CAD build for the part. Positions are in the model's coordinates, mm. A direction names the side the tool comes from. Round coordinates to 2 decimals unless told otherwise and drop trailing zeros. Loops run counter-clockwise (first coordinate to the right, second up) from the corner with the lowest first, then second, coordinate; pieces in that order, holes last. Notation, with made-up numbers: (37, 84) - (60, 84) arc R14 ccw to (60, 105) - close; hole circle Ø7 at (-9, 60). An arc over 180 degrees is marked (long way). One line per question, with ' | ' between items.
```python
from build123d import *

# Parameters (mm, degrees)
SKETCH2_W           = 75
SKETCH2_H           = 48
BOSS_EXTRUDE1_DEPTH = 7.75
CUT_EXTRUDE4_DEPTH  = 12.5
SKETCH12_W          = 50
SKETCH12_H          = 38
CUT_EXTRUDE5_DEPTH  = 7.75
SKETCH13_R          = 0.625
CUT_EXTRUDE6_DEPTH  = 47.006113724
FILLET4_R           = 3
SKETCH14_W          = 2
SKETCH14_H          = 5
BOSS_EXTRUDE2_DEPTH = 2
SKETCH16_R          = 1.25
CUT_EXTRUDE9_DEPTH  = 1
SKETCH18_R          = 5
CUT_EXTRUDE10_DEPTH = 3
SKETCH19_R          = 7.5
CUT_EXTRUDE11_DEPTH = 0.5


with BuildPart() as part:
    # Sketch2 → Boss-Extrude1 (new, symmetric)
    with BuildSketch(Plane.XY):
        with Locations((0, 1.5)):
            Rectangle(SKETCH2_W, SKETCH2_H)
    extrude(amount=BOSS_EXTRUDE1_DEPTH, both=True)

    # Sketch11 → Cut-Extrude4 (cut)
    with BuildSketch(Plane(origin=(0, 0, -7.75), x_dir=(-1, 0, 0), z_dir=(0, 0, -1))):
        Polygon((-35, 22.5), (35, 22.5), (30, -22.5), (-30, -22.5), align=None)
    extrude(amount=-CUT_EXTRUDE4_DEPTH, mode=Mode.SUBTRACT)

    # Sketch12 → Cut-Extrude5 (cut, symmetric)
    with BuildSketch(Plane.XY):
        with Locations((0, 6.5)):
            Rectangle(SKETCH12_W, SKETCH12_H)
    extrude(amount=CUT_EXTRUDE5_DEPTH, both=True, mode=Mode.SUBTRACT)

    # Sketch13 → Cut-Extrude6 (cut, through all)
    with BuildSketch(Plane.XY):
        with Locations(Location((13, -20, 0), (0, 0, 180))):
            Circle(SKETCH13_R)
        with Locations(Location((-13, -20, 0), (0, 0, 180))):
            Circle(SKETCH13_R)
        with BuildLine():
            Line((-5, -22.5), (5, -22.5))
            ThreePointArc((5, -22.5), (0, -17.5), (-5, -22.5))
        make_face()
    extrude(amount=CUT_EXTRUDE6_DEPTH, mode=Mode.SUBTRACT)

    # Fillet4
    fillet4_edges = [part.edges().sort_by_distance(p)[0] for p in [
        (0, -17.5, 7.75),
        (37.5, 1.5, 7.75),
        (25, 6.5, 7.75),
        (-25, 6.5, 7.75),
        (-37.5, 1.5, 7.75),
        (25, 25.5, 0),
        (-25, 25.5, 0),
        (-37.5, 25.5, 0),
        (37.5, 25.5, 0),
        (31.25, 25.5, 7.75),
        (-31.25, 25.5, 7.75),
        (-37.5, -22.5, 0),
        (37.5, -22.5, 0),
    ]]
    fillet(fillet4_edges, radius=FILLET4_R - 0.0001)  # a hair under: the kernel refuses the full size

    # Sketch14 → Boss-Extrude2 (add)
    with BuildSketch(Plane(origin=(0, 0, -7.75), x_dir=(-1, 0, 0), z_dir=(0, 0, -1))):
        with Locations((-36.5, -14)):
            Rectangle(SKETCH14_W, SKETCH14_H)
        with Locations((36.5, -14)):
            Rectangle(SKETCH14_W, SKETCH14_H)
    extrude(amount=BOSS_EXTRUDE2_DEPTH)

    # Sketch16 → Cut-Extrude9 (cut)
    with BuildSketch(Plane.XY.offset(7.75)):
        with Locations((-13, -20)):
            Circle(SKETCH16_R)
        with Locations(Location((13, -20, 0), (0, 0, 180))):
            Circle(SKETCH16_R)
    extrude(amount=-CUT_EXTRUDE9_DEPTH, mode=Mode.SUBTRACT)

    # Sketch18 → Cut-Extrude10 (cut)
    with BuildSketch(Plane(origin=(37.5, 0, 0), x_dir=(0, 0, -1), z_dir=(1, 0, 0))):
        with Locations((7.75, 10)):
            Circle(SKETCH18_R)
    cut_extrude10 = extrude(amount=-CUT_EXTRUDE10_DEPTH, mode=Mode.SUBTRACT)

    # Sketch19 → Cut-Extrude11 (cut, symmetric)
    with BuildSketch(Plane(origin=(36, 0, 0), x_dir=(0, 0, -1), z_dir=(1, 0, 0))):
        with Locations((7.75, 10)):
            Circle(SKETCH19_R)
    cut_extrude11 = extrude(amount=CUT_EXTRUDE11_DEPTH, both=True, mode=Mode.SUBTRACT)

    # Mirror1: Cut-Extrude10, Cut-Extrude11 across plane
    add(cut_extrude10.mirror(Plane(origin=(0, 0, 0), x_dir=(0, 0, 1), z_dir=(1, 0, 0))), mode=Mode.SUBTRACT)
    add(cut_extrude11.mirror(Plane(origin=(0, 0, 0), x_dir=(0, 0, 1), z_dir=(1, 0, 0))), mode=Mode.SUBTRACT)


solid = part.part
```
(1) Drop flat-ended pins along their axis: P1, Ø2, axis at x = 36, z = -9, coming from the -Y side; P2, Ø2, axis at x = 13, y = -20, coming from the -Z side; P3, Ø2, axis at x = -36, z = -8.5, coming from the -Y side. Give the stop position or say it passes through.
Results found:
P1: stops at y = -16.5 | P2: stops at z = 4.75 | P3: stops at y = -22.38
(2) Tool access for faces 1 (the face through (-36.5, 10, -2)), 2 (the face through (-25.9, 24.64, -1.59)), 3 (the face through (-13.27, -21.22, 7.26)), 4 (the face through (37.01, 10.11, -2.75)), 5 (the face through (-35.01, 10.11, -2.75)): list every direction of +Z, -Z, +X, -X, +Y, -Y with a clear straight run to the whole face (end or side of a thin tool).
Results found:
face 1: -Z | face 2: +Z, -Z, +Y | face 3: +Z | face 4: -Z, +X | face 5: -Z, -X
(3) Two-plate mould, pull along Y, no slides. Class faces 6 (the face through (-36, -11.5, -9)), 7 (the face through (37.5, 1, -1)), 8 (the face through (13, -21, 6.75)): released by +Y, released by -Y, zero draft, split by the parting line, or undercut.
Results found:
face 6: released by +Y | face 7: zero draft | face 8: undercut
(4) Probe L1, parallel to Z at x = 29, y = -19.5; L2, parallel to X at y = 6.5, z = -1.75; L3, parallel to X at y = 21.5, z = 4.25. List the from-to ranges inside material, lowest first.
Results found:
L1: z = 4.75 to 7.75 | L2: x = -37.5 to -36.5, -35.5 to -33.22, 33.22 to 35.5, 36.5 to 37.5 | L3: x = -37.5 to -34.89, 34.89 to 37.5
(5) Cut at B-B, the plane x = 32.5. Write the cut outline in (y, z).
Results found:
outline: (-22.5, -7.75) - (0, -7.75) - (0, 4.75) - (22.5, 4.75) - (22.5, -7.75) - (25.5, -7.75) - (25.5, 4.75) arc R3 ccw to (22.5, 7.75) - (-22.5, 7.75) - close
